Autodesk Inventor part; units mm, degrees
ref_plane "Work Plane1" through (0, 0, 0) normal (0, 0.2308893, 0.97298) x (1, 0, 0)
ref_plane "YZ Plane" through (0, 0, 0) normal (1, 0, 0) x (0, 1, 0)
ref_plane "XZ Plane" through (0, 0, 0) normal (0, 1, 0) x (-1, 0, 0)
sketch "Sketch1" plane through (0, 0, 0) normal (1, 0, 0) x (0, 1, 0)
  line L0 (0, 0) -> (67.821, 0)
  line L1 (67.821, 0) -> (67.821, -16.094)
  line L2 (67.821, -16.094) -> (0, -16.094)
  line L3 (0, -16.094) -> (0, 0)
  line L4 (67.821, -16.094) -> (0, 0)
  dimension "d0" = 67.821
  dimension "d1" = 16.094
ref_plane "Work Plane1" through (0, 0, 0) normal (0, 0.2308893, 0.97298) x (1, 0, 0)
sketch "Sketch4" plane through (0, 0, 0) normal (0, 0.2308893, 0.97298) x (1, 0, 0)
  line L0 (0, 0) -> (-10, 0)
  line L1 (-10, 0) -> (-10, -40)
  line L2 (-10, -40) -> (0, -40)
  line L3 (0, -40) -> (0, 0)
  dimension "d16" = 40
  dimension "d17" = 10
extrude "Extrusion4" add sketch "Sketch4" along normal blind 20
fillet "Fillet3" radius 2.5 8 edges at (0, -14.8418, 24.0774) (-10, -14.8418, 24.0774) (-5, 4.6178, 19.4596) (-10, 2.3089, 9.7298) (0, 2.3089, 9.7298) (0, -36.6103, 18.9654) (-5, -34.3014, 28.6952) (-10, -36.6103, 18.9654)
shell "Shell2" thickness 1 removed faces 0
sketch "Sketch5" plane through (-7.5, -38.9192, 9.2356) normal (0, -0.97298, 0.2308893) x (1, 0, 0)
  line L0 (0, 0) -> (0, 17.5)
  line L1 (0, 0) -> (5, 0)
  line L2 (5, 17.5) -> (5, 0)
  line L3 (0, 17.5) -> (5, 17.5)
  circle A0 centre (2.5, 14.5) radius 1.5
  point P0 (7.5, 0)
  point P1 (2.5, 17.5)
  dimension "d22" = 3
  dimension "d23" = 3
extrude "Extrusion5" cut sketch "Sketch5" against normal blind 2 contours A0
fillet "Fillet4" radius 0.5 2 edges at (-6.5, -34.5983, 23.1129) (-6.5, -35.5713, 23.3438)
sketch "Sketch6" plane through (0, -36.4868, 8.6583) normal (1, 0, 0) x (0, -0.2308893, -0.97298)
  line L0 (-17.5, 35) -> (0, 35)
  line L1 (-17.5, 0) -> (-17.5, 35)
  line L2 (0, 0) -> (-17.5, 0)
  line L3 (0, 0) -> (0, 35)
  point P0 (0, 37.5)
  dimension "d27" = 35
  dimension "d28" = 17.5
sketch "Sketch7" plane through (-10, -36.4868, 8.6583) normal (-1, 0, 0) x (0, 0.2308893, 0.97298)
  line L0 (0, -2.5) -> (17.5, -2.5)
  line L1 (20, 0) -> (20, 35)
  line L2 (20, -2.5) -> (6.9383, -2.5)
  line L3 (7.5, 6.273) -> (20, 6.273)
  line L4 (20, 6.273) -> (20, -2.5)
  line L5 (0, -2.5) -> (20, -2.5)
  line L6 (12.5, -2.5) -> (16.5, -2.5)
  line L7 (20, 6.273) -> (20, -2.5)
  line L8 (20, -2.5) -> (20, 16.6364)
  line L9 (20, 35) -> (20, 0)
  line L10 (7.5, 6.273) -> (7.5, -2.5)
  circle A0 centre (7.5, 6.273) radius 0.75
  point P0 (0, 37.5)
  dimension "d29" = 12.5
  dimension "d30" = 8.773
  dimension "d31" = 1.5
extrude "Extrusion6" add sketch "Sketch7" against normal blind 10 contours A0 L3 L10 | L10 L3 A0
properties part number "caja de los actuadores"
Design review of the part built by this model. Coordinates are the model's own, in mm. A direction names the side the tool comes from. Coordinates: 2 decimals unless noted, no trailing zeros. Order: outer loops, then holes, each group sorted by start corner. A loop starts at its lowest first (then second) coordinate and runs counter-clockwise, first axis right, second up. Notation, with made-up numbers: (66.5, 15) - (110.5, 15) arc R25 ccw to (110.5, 40) - close; hole circle Ø5 at (79, 61.25). An arc over 180 degrees is marked (long way). Put each result on its own line as item: value.
1) Insertion check: P1, Ø1, axis at x = -8, z = 18.5, coming from the +Y side; P2, Ø1.5, axis at x = -3.5, y = -33.5, coming from the -Z side; P3, Ø2, axis at y = -11.5, z = 22, coming from the +X side. Each pin has a flat end and moves straight along its axis. Give the tip position at first contact, or say it passes through.
Response values:
P1: stops at y = 4.05
P2: stops at z = 7.77
P3: stops at x = -0.01
2) Take a section at A-A, the plane x = -2. Give the boundary of the cut face in (y, z).
Response values:
outline: (-38.87, 9.22) - (-0.05, 0.01) - (3.99, 17.04) arc R2.45 ccw to (2.17, 19.99) - (-31.88, 28.07) arc R2.45 ccw to (-34.83, 26.25) - close; circle Ø1.5 at (-28.65, 14.51); hole (-37.63, 9.96) - (-0.83, 1.22) - (2.98, 17.28) arc R1.41 ccw to (1.93, 18.98) - (-32.12, 27.06) arc R1.41 ccw to (-33.82, 26.01) - close
3) Wall thickness on L1, parallel to Y at x = -2.75, z = 14.25; L2, parallel to Y at x = -6.75, z = 14; L3, parallel to X at y = -25.5, z = 10.25: over which ranges is each line inside the solid? List them lowest first. Write a range as from..to.
Response values:
L1: y = -37.73..-36.7, -29.36..-27.95, 2.35..3.38
L2: y = -37.79..-36.76, -29.2..-28.1, 2.29..3.32
L3: x = -10..-9, -1..0
4) The part is to be moulded in two halves that separate along Y. For faces 3 (the face through (-4.96, -33.73, 27.83)), 4 (the face through (-1.45, -14.93, 22.63)), 5 (the face through (-4.96, -33.22, 26.97)), 6 (the face through (-5.07, -19.187, 4.553)), say which applies: released by +Y, released by -Y, zero draft, split by the parting line, or undercut.
Response values:
face 3: split by the parting line
face 4: undercut
face 5: undercut
face 6: released by -Y
5) Tool access review of faces 1 (the face through (-1, -18, 14)), 2 (the face through (-0.752, -14.768, 23.327)): name each direction out of +Z, -Z, +X, -X, +Y, -Y from which nothing blocks a thin tool from reaching the whole face with its end or side.
Response values:
face 1: none
face 2: +Z, +X, +Y
